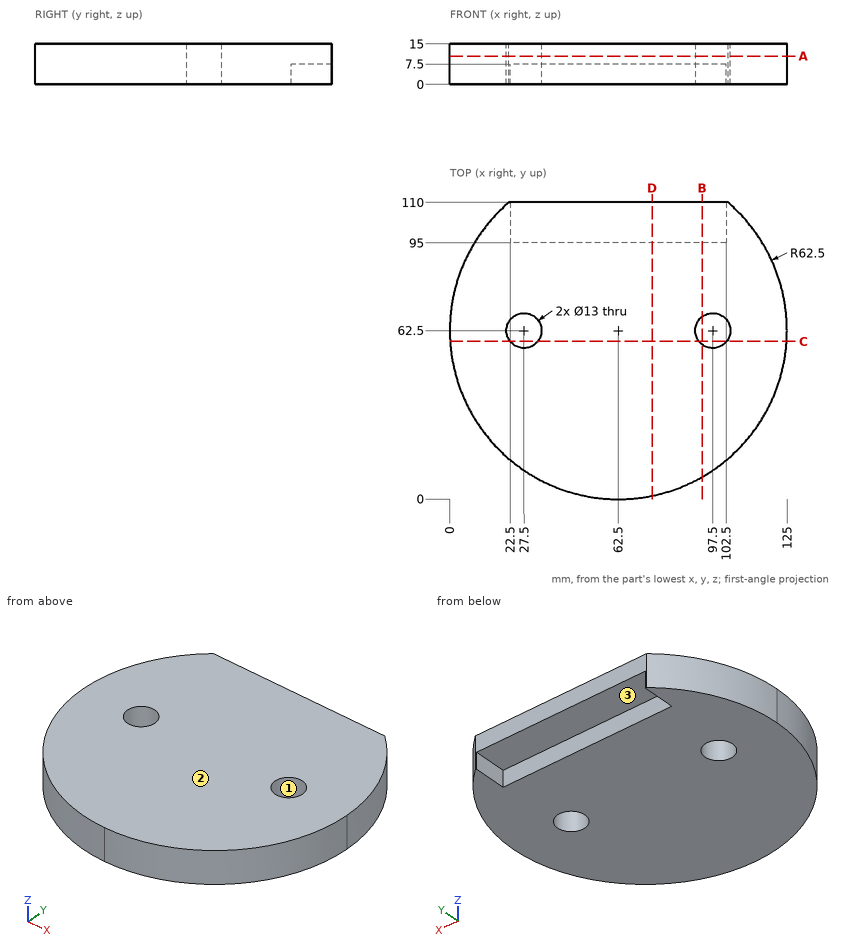
Study the drawing (mm; zero at the part's minimum x, y, z) and answer. Give positions to 0.01 mm unless a question says otherwise; leave off trailing zeros. Loops run counter-clockwise (first coordinate to the right, second up) from the corner with the lowest first, then second, coordinate; pieces in that order, holes last. Notation, with made-up numbers: (-30.5, 88) - (8.5, 88) arc R15 ccw to (8.5, 115) - close; hole circle Ø1 at (86.5, 79). An arc over 180 degrees is marked (long way). Use CSV: the item, a comma, the result in double quotes. Start each with the question number.
(1) Find the intervals of material crossed by L1, parallel to X at y = 68, z = 12.75 (1 decimal); L2, parallel to X at y = 64, z = 3.25 (1 decimal); L3, parallel to Y at x = 28, z = 9.5 (1 decimal), in increasing order.
(2) Find section C-C, the plane y = 58.5. Determine the outline of the cut face in (x, z).
(3) Find section A-A, the plane z = 10.5. Determine the outline of the cut face in (x, y).
(4) Determine the mould class of the marked faces 1, 2 and 3 for opening direction X: released by +X, released by -X, zero draft, split by the parting line, or undercut.
(5) Find section D-D, the plane x = 75. Determine the outline of the cut face in (y, z), plus the area to 3 significant figures.
(6) Find section B-B, the plane x = 93.5. Determine the outline of the cut face in (y, z).
(7) Each of these flat-tipped pins is pushed along its axis until it touches: pin 1 (12 mm diameter, centred on x = 63, y = 105, fed in from -Z); pin 2 (6 mm diameter, centred on y = 29.5, z = 9, fed in from -X); pin 3 (6 mm diameter, centred on y = 103, z = 2.5, fed in from -X); pin 4 (10.5 mm diameter, centred on x = 27.5, y = 62.5, fed in from +Z). Where does it stop, or does it pass through?
Results found:
1,L1,"0.2 to 24, 31 to 94, 101 to 124.8"
1,L2,"0 to 21.2, 33.8 to 91.2, 103.8 to 125"
1,L3,"10.4 to 56, 69 to 110"
2,outline,"(0.13, 0) - (22.38, 0) - (22.38, 15) - (0.13, 15) - close; (32.62, 0) - (92.38, 0) - (92.38, 15) - (32.62, 15) - close; (102.62, 0) - (124.87, 0) - (124.87, 15) - (102.62, 15) - close"
3,outline,"(21.88, 110) arc R62.5 ccw (long way) to (103.12, 110) - close; hole circle Ø13 at (27.5, 62.5); hole circle Ø13 at (97.5, 62.5)"
4,face 1,"undercut"
4,face 2,"zero draft"
4,face 3,"undercut"
5,outline,"(1.26, 0) - (95, 0) - (95, 7.5) - (110, 7.5) - (110, 15) - (1.26, 15) - close"
5,area,"1,520 mm^2"
6,outline,"(8.23, 0) - (57.38, 0) - (57.38, 15) - (8.23, 15) - close; (67.62, 0) - (95, 0) - (95, 7.5) - (110, 7.5) - (110, 15) - (67.62, 15) - close"
7,pin 1,"z = 7.5"
7,pin 2,"x = 7.67"
7,pin 3,"x = 12.5"
7,pin 4,"through"
